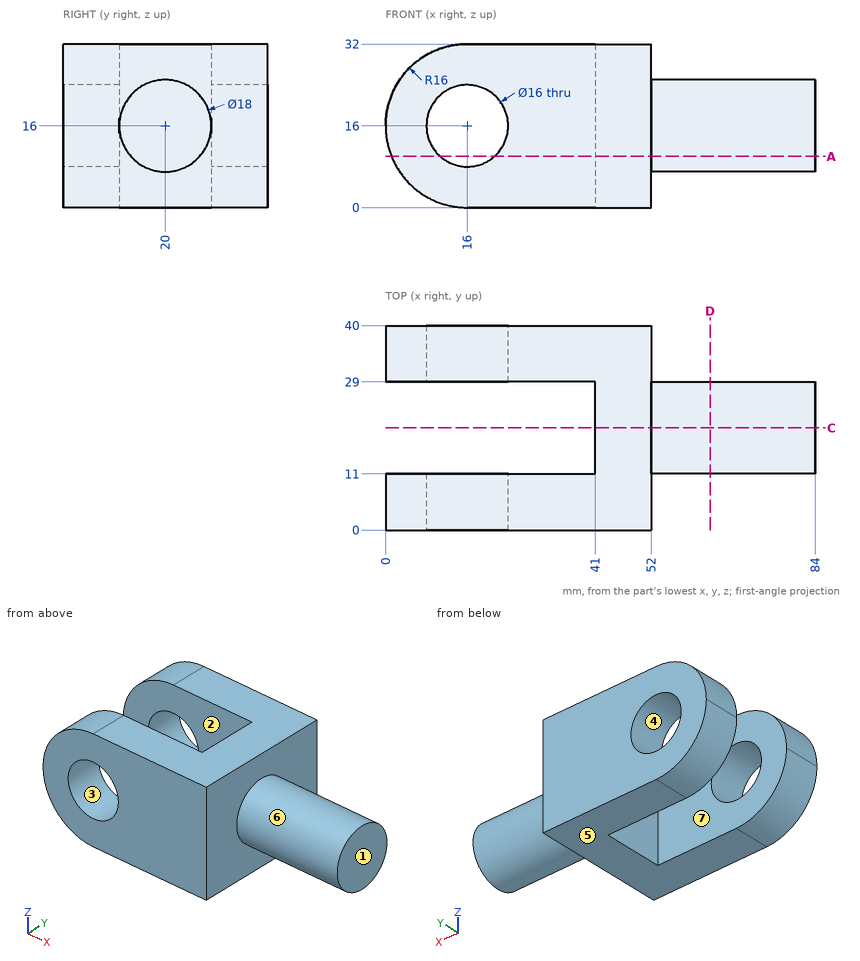
Input: dimensioned drawing with shaded views. Units: mm. Origin: part minimum x, y, z. A direction names the side the tool comes from. Give positions to 0.01 mm unless a question says otherwise; leave off trailing zeros. Write each loop counter-clockwise with the first axis right and the second up, starting at its lowest first coordinate (ties: lowest second). Pieces come first, ordered by that corner, then holes.
1. Line query: probe 1 along Z at (x, y) = (16, 4); probe 2 along Y at (x, z) = (39, 13.5); probe 3 along X at (y, z) = (14, 30). Output: solid intervals per line, ascending.
2. Section query C-C, the plane y = 20. Return loops of the section in (x, z), then the cut area to 3 significant figures.
3. Section query A-A, the plane z = 10. Return loops of the section in (x, y), then the cut area to 3 significant figures.
4. Draft query along X for the marked faces 1, 2, 3 and 4. Return one class per face: released by +X, released by -X, zero draft, split by the parting line, or undercut.
5. Section query D-D, the plane x = 63.5. Return loops of the section in (y, z).
6. Reachability of the marked faces 5, 6 and 7 from +Z, -Z, +X, -X, +Y, -Y: full face, straight path, thin tool, end or side. Return the list, or none.
7. Pin query (flat end, axial travel): P1, Ø5.5, axis at y = 24, z = 19.5, coming from the -X side; P2, Ø4, axis at y = 10.5, z = 5.5, coming from the +X side; P3, Ø5, axis at x = 68, z = 6, coming from the +Y side (3 decimals). Return the tip coordinate at first contact, or that it passes through.
Computed:
1. probe 1: z = 0 to 8, 24 to 32
1. probe 2: y = 0 to 11, 29 to 40
1. probe 3: x = 41 to 52
2. outline: (41, 0) - (52, 0) - (52, 7) - (84, 7) - (84, 25) - (52, 25) - (52, 32) - (41, 32) - close
2. area: 928 mm2
3. outline: (1.17, 0) - (10.71, 0) - (10.71, 11) - (1.17, 11) - close; (1.17, 29) - (10.71, 29) - (10.71, 40) - (1.17, 40) - close; (21.29, 0) - (52, 0) - (52, 13.29) - (84, 13.29) - (84, 26.71) - (52, 26.71) - (52, 40) - (21.29, 40) - (21.29, 29) - (41, 29) - (41, 11) - (21.29, 11) - close
3. area: 1,510 mm2
4. face 1: released by +X
4. face 2: zero draft
4. face 3: undercut
4. face 4: undercut
5. outline: circle Ø18 at (20, 16)
6. face 5: -Z, +X, -X, +Y, -Y
6. face 6: +X
6. face 7: +Z, -Z, -X
7. P1: stops at x = 41
7. P2: stops at x = 52
7. P3: stops at y = 24.975
